Verification items for the finished model (mm, model axes). Face numbers are marked on the shaded views. A direction names the side the tool comes from. Round coordinates to 2 decimals unless told otherwise and drop trailing zeros. Loops run counter-clockwise (first coordinate to the right, second up) from the corner with the lowest first, then second, coordinate; pieces in that order, holes last. Notation, with made-up numbers: (68, 75.5) - (95, 75.5) arc R33 ccw to (95, 110.5) - close; hole circle Ø6 at (-5, 66). An arc over 180 degrees is marked (long way). Use CSV: the item, a comma, the result in double quotes.
```python
from build123d import *

# Parameters (mm, degrees)
BOSS_EXTRUDE1_DEPTH     = 35
CONVERT_SOLID1_DEPTH    = 35
CUT_EXTRUDE1_DEPTH      = 68.63261331
CUT_EXTRUDE1_DEPTH_BACK = 7.5
SKETCH2_R               = 1.5


# Read off the part's stored shape, not the designer's step: Convert-Solid1
with BuildPart() as part:
    # Sketch1 → Boss-Extrude1 (new body)
    with BuildSketch(Plane.XY):
        with BuildLine():
            Line((0, 0), (30, 0))
            ThreePointArc((30, 0), (34.770067359, 1.975826594), (36.745893953, 6.745893953))
            Line((36.745893953, 6.745893953), (36.745893953, 31.745893953))
            ThreePointArc((36.745893953, 31.745893953), (34.768864726, 36.518864726), (29.995893953, 38.495893953))
            Line((29.995893953, 38.495893953), (-0.004106047, 38.495893953))
            Line((-0.004106047, 38.495893953), (-0.004106047, 36.995893953))
            Line((-0.004106047, 36.995893953), (29.995893953, 36.995893953))
            ThreePointArc((29.995893953, 36.995893953), (33.708204554, 35.458204554), (35.245893953, 31.745893953))
            Line((35.245893953, 31.745893953), (35.245893953, 6.75))
            ThreePointArc((35.245893953, 6.75), (33.708204554, 3.037689399), (29.995893953, 1.5))
            Line((29.995893953, 1.5), (0, 1.5))
            Line((0, 1.5), (0, 0))
        make_face()
    extrude(amount=BOSS_EXTRUDE1_DEPTH)

    # Convert-Solid1 outline → Convert-Solid1 (add)
    with BuildSketch(Plane.XY):
        with BuildLine():
            Line((29.995893953, 36.995893953), (-0.004106047, 36.995893953))
            Line((-0.004106047, 36.995893953), (-0.004106047, 36.495893953))
            Line((-0.004106047, 36.495893953), (29.995893953, 36.495893953))
            ThreePointArc((29.995893953, 36.495893953), (33.354651163, 35.104651163), (34.745893953, 31.745893953))
            Line((34.745893953, 31.745893953), (34.745893953, 6.745893953))
            ThreePointArc((34.745893953, 6.745893953), (33.355853797, 3.390040156), (30, 2))
            Line((30, 2), (0, 2))
            Line((0, 2), (0, 1.5))
            Line((0, 1.5), (29.995893953, 1.5))
            ThreePointArc((29.995893953, 1.5), (33.708204554, 3.037689399), (35.245893953, 6.75))
            Line((35.245893953, 6.75), (35.245893953, 31.745893953))
            ThreePointArc((35.245893953, 31.745893953), (33.708204554, 35.458204554), (29.995893953, 36.995893953))
        make_face()
    extrude(amount=CONVERT_SOLID1_DEPTH)

    # Sketch2 → Cut-Extrude1 (cut, two sides: drawn at the far end of the back side and taken through both)
    with BuildSketch(Plane(origin=(54.180486852, 36.495893953, 17.5), x_dir=(0, 0, 1), z_dir=(0, -1, 0)).offset(-CUT_EXTRUDE1_DEPTH_BACK)):
        with Locations(Location((11.5, 34.184592899, 0), (0, 0, 270))):
            Circle(SKETCH2_R)
        with Locations(Location((-11.5, 34.184592899, 0), (0, 0, 270))):
            Circle(SKETCH2_R)
    extrude(amount=CUT_EXTRUDE1_DEPTH + CUT_EXTRUDE1_DEPTH_BACK, mode=Mode.SUBTRACT)


solid = part.part
```
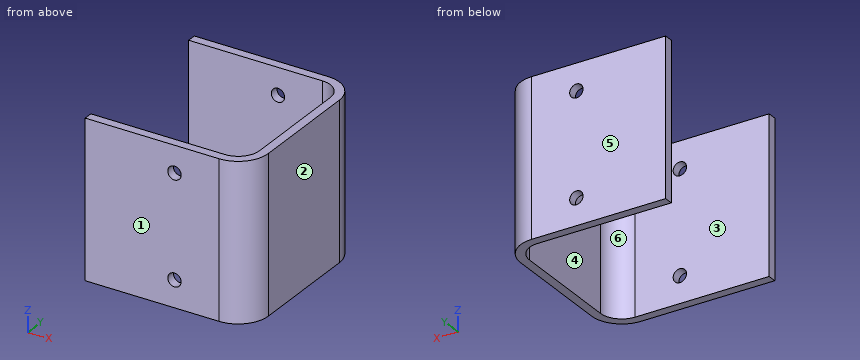
1) Access from +Z, -Z, +X, -X, +Y, -Y to the whole of each face (thin tool, end or side, straight path). Record for the marked faces 5 and 6.
Returned:
face 5,"+Z, -Z, +X, -X, +Y"
face 6,"+Z, -Z, -X"
2) Cross-section at B-B, the plane z = 29. Record the cut outline in (x, y), then the cut area to 3 significant figures.
Returned:
outline,"(0, 0) - (18.5, 0) - (18.5, 2) - (0, 2) - close; (0, 36.5) - (18.5, 36.5) - (18.5, 38.5) - (0, 38.5) - close; (21.5, 0) - (30, 0) arc R6.75 ccw to (36.75, 6.75) - (36.75, 31.75) arc R6.75 ccw to (30, 38.5) - (21.5, 38.5) - (21.5, 36.5) - (30, 36.5) arc R4.75 cw to (34.75, 31.75) - (34.75, 6.75) arc R4.75 cw to (30, 2) - (21.5, 2) - close"
area,"194 mm²"
3) Thickness scan on probe 1 along Y at (x, z) = (13, 29); probe 2 along X at (y, z) = (20.5, 29.5); probe 3 along X at (y, z) = (37, 6). Record the ranges inside material, lowest first. Write a range as [from, to].
Returned:
probe 1,"y = [0, 2], [36.5, 38.5]"
probe 2,"x = [34.75, 36.75]"
probe 3,"x = [0, 18.5], [21.5, 34.23]"
4) Cross-section at A-A, the plane x = 28. Record the cut outline in (y, z), then the cut area to 3 significant figures.
Returned:
outline,"(0, 0) - (2, 0) - (2, 35) - (0, 35) - close; (36.5, 0) - (38.5, 0) - (38.5, 35) - (36.5, 35) - close"
area,"140 mm²"
5) Cross-section at C-C, the plane z = 11.5. Record the cut outline in (x, y).
Returned:
outline,"(0, 0) - (30, 0) arc R6.75 ccw to (36.75, 6.75) - (36.75, 31.75) arc R6.75 ccw to (30, 38.5) - (0, 38.5) - (0, 36.5) - (30, 36.5) arc R4.75 cw to (34.75, 31.75) - (34.75, 6.75) arc R4.75 cw to (30, 2) - (0, 2) - close"
6) Cross-section at D-D, the plane y = 17.5. Record the cut outline in (x, z), then the cut area to 3 significant figures.
Returned:
outline,"(34.75, 0) - (36.75, 0) - (36.75, 35) - (34.75, 35) - close"
area,"70.0 mm²"
7) Mould release check, pull along Y, two halves, no side actions. Record for the marked faces 1, 2, 3 and 4: +Y half, -Y half, draft (parallel to the pull), parting line (faces both ways), or undercut.
Returned:
face 1,"-Y half"
face 2,"draft"
face 3,"undercut"
face 4,"undercut"
8) Gauge pin test, flat ends, axial feed: pin 1 Ø10 at (y, z) = (12, 12.5) entering from -X; pin 2 Ø12 at (y, z) = (28.5, 4.5) entering from -X; pin 3 Ø4 at (x, z) = (31.5, 30.5) entering from +Y; pin 4 Ø1 at (y, z) = (1, 14.5) entering from -X. Record the tip position at first contact, or that the pin passes through.
Returned:
pin 1,"stops at x = 34.75"
pin 2,"stops at x = 33.87"
pin 3,"stops at y = 38.5"
pin 4,"stops at x = 0"
